```python
from build123d import *

# Parameters (mm, degrees)
SKETCH1_W           = 22.5
SKETCH1_H           = 12
BOSS_EXTRUDE1_DEPTH = 21
SKETCH2_W           = 32.5
SKETCH2_H           = 12
BOSS_EXTRUDE2_DEPTH = 3
SKETCH3_W           = 22.5
SKETCH3_H           = 12
BOSS_EXTRUDE6_DEPTH = 4
SKETCH5_W           = 12
SKETCH5_H           = 12
BOSS_EXTRUDE7_DEPTH = 5
SKETCH6_R           = 3.5
BOSS_EXTRUDE8_DEPTH = 5
SKETCH7_R           = 1.2
CUT_EXTRUDE1_DEPTH  = 5
FILLET3_R           = 3
FILLET4_R           = 1
FILLET5_R           = 1
FILLET6_R           = 1
FILLET7_R           = 1
FILLET8_R           = 1
FILLET9_R           = 1
FILLET10_R          = 0.2
SKETCH14_R          = 2.1
CUT_EXTRUDE4_DEPTH  = 5
SKETCH13_R          = 2.1
CUT_EXTRUDE5_DEPTH  = 5
FILLET11_R          = 1


with BuildPart() as part:
    # Sketch1 → Boss-Extrude1 (new body)
    with BuildSketch(Plane.XY):
        Rectangle(SKETCH1_W, SKETCH1_H)
    extrude(amount=BOSS_EXTRUDE1_DEPTH)

    # Sketch2 → Boss-Extrude2 (add)
    with BuildSketch(Plane.XY):
        Rectangle(SKETCH2_W, SKETCH2_H)
    extrude(amount=-BOSS_EXTRUDE2_DEPTH)

    # Sketch3 → Boss-Extrude6 (add)
    with BuildSketch(Plane(origin=(0, 0, -3), x_dir=(-1, 0, 0), z_dir=(0, 0, -1))):
        Rectangle(SKETCH3_W, SKETCH3_H)
    extrude(amount=BOSS_EXTRUDE6_DEPTH)

    # Sketch5 → Boss-Extrude7 (add)
    with BuildSketch(Plane(origin=(0, 0, -7), x_dir=(-1, 0, 0), z_dir=(0, 0, -1))):
        with Locations((-5.25, 0)):
            Rectangle(SKETCH5_W, SKETCH5_H)
    extrude(amount=BOSS_EXTRUDE7_DEPTH)

    # Sketch6 → Boss-Extrude8 (add)
    with BuildSketch(Plane(origin=(0, 0, -12), x_dir=(-1, 0, 0), z_dir=(0, 0, -1))):
        with Locations(Location((-5.25, 0, 0), (0, 0, 180))):
            Circle(SKETCH6_R)
    extrude(amount=BOSS_EXTRUDE8_DEPTH)

    # Sketch7 → Cut-Extrude1 (cut)
    with BuildSketch(Plane(origin=(0, 0, -17), x_dir=(-1, 0, 0), z_dir=(0, 0, -1))):
        with Locations((-5.25, 0)):
            Circle(SKETCH7_R)
    extrude(amount=-CUT_EXTRUDE1_DEPTH, mode=Mode.SUBTRACT)

    # Fillet3
    fillet3_edges = [part.edges().sort_by_distance(p)[0] for p in [
        (-11.25, 0, -7),
    ]]
    fillet(fillet3_edges, radius=FILLET3_R)

    # Fillet4
    fillet4_edges = [part.edges().sort_by_distance(p)[0] for p in [
        (11.25, 0, -12),
    ]]
    fillet(fillet4_edges, radius=FILLET4_R)

    # Fillet5
    fillet5_edges = [part.edges().sort_by_distance(p)[0] for p in [
        (-0.75, 0, -12),
    ]]
    fillet(fillet5_edges, radius=FILLET5_R)

    # Fillet6
    fillet6_edges = [part.edges().sort_by_distance(p)[0] for p in [
        (11.25, -6, -7),
        (10.957106781, -6, -11.707106781),
        (-0.75, -6, -9),
        (-0.457106781, -6, -11.707106781),
        (5.25, -6, -12),
    ]]
    fillet(fillet6_edges, radius=FILLET6_R)

    # Fillet7
    fillet7_edges = [part.edges().sort_by_distance(p)[0] for p in [
        (11.25, 6, -7),
        (10.957106781, 6, -11.707106781),
        (-0.75, 6, -9),
        (-0.457106781, 6, -11.707106781),
        (5.25, 6, -12),
    ]]
    fillet(fillet7_edges, radius=FILLET7_R)

    # Fillet8
    fillet8_edges = [part.edges().sort_by_distance(p)[0] for p in [
        (-11.25, 6, -3.5),
        (-10.371320344, 6, -6.121320344),
        (-4, 6, -7),
    ]]
    fillet(fillet8_edges, radius=FILLET8_R)

    # Fillet9
    fillet9_edges = [part.edges().sort_by_distance(p)[0] for p in [
        (-11.25, -6, -3.5),
        (-10.371320344, -6, -6.121320344),
        (-4, -6, -7),
    ]]
    fillet(fillet9_edges, radius=FILLET9_R)

    # Fillet10
    fillet10_edges = [part.edges().sort_by_distance(p)[0] for p in [
        (1.75, 0, -17),
    ]]
    fillet(fillet10_edges, radius=FILLET10_R)

    # Sketch14 → Cut-Extrude4 (cut)
    with BuildSketch(Plane(origin=(0, 0, -3), x_dir=(-1, 0, 0), z_dir=(0, 0, -1))):
        with Locations((15, 0)):
            Circle(SKETCH14_R)
    extrude(amount=-CUT_EXTRUDE4_DEPTH, mode=Mode.SUBTRACT)

    # Sketch13 → Cut-Extrude5 (cut)
    with BuildSketch(Plane(origin=(0, 0, -3), x_dir=(-1, 0, 0), z_dir=(0, 0, -1))):
        with Locations((-15, 0)):
            Circle(SKETCH13_R)
    extrude(amount=-CUT_EXTRUDE5_DEPTH, mode=Mode.SUBTRACT)

    # Fillet11
    fillet11_edges = [part.edges().sort_by_distance(p)[0] for p in [
        (-16.25, -6, -1.5),
        (-16.25, 6, -1.5),
        (16.25, -6, -1.5),
        (16.25, 6, -1.5),
    ]]
    fillet(fillet11_edges, radius=FILLET11_R)


solid = part.part
```
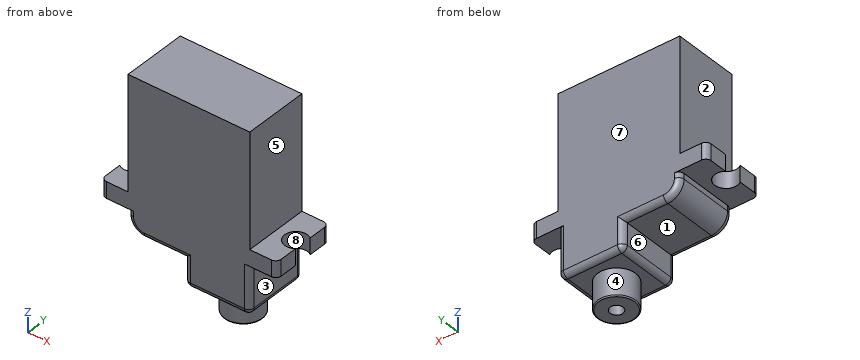
The listing builds one solid part. Answer for the finished solid, in the listing's coordinates (mm). Face numbers are marked on the shaded views. A direction names the side the tool comes from. Give positions to 0.01 mm unless a question says otherwise; leave off trailing zeros. Write each loop counter-clockwise with the first axis right and the second up, starting at its lowest first coordinate (ties: lowest second). Pieces come first, ordered by that corner, then holes. Notation, with made-up numbers: (-30.75, 40.25) -> (-19.75, 40.25) arc R18 ccw to (-19.75, 59.25) -> close; hole circle Ø3 at (45, -15). An arc over 180 degrees is marked (long way). Write item = value, one per line. Start each with the question number.
1) Straight lines are drawn through the part: line 1 along Y through (x, z) = (15, -0.9); line 2 along Z through (x, y) = (12.5, -3.25); line 3 along X through (y, z) = (0, -1.6). For each, find the intervals that lie inside material, in ascending order.
2) Each of these flat-tipped pins is pushed along its axis until it touches: pin 1 (1 mm diameter, centred on y = 1, z = 4.5, fed in from -X); pin 2 (6.5 mm diameter, centred on x = 13.5, y = 0, fed in from -Z); pin 3 (5 mm diameter, centred on x = -13, y = 2.5, fed in from -Z). Where does it stop, or does it pass through?
3) The part is cut by section D-D, the plane x = -5.5. Determine the outline of the cut face in (y, z).
4) The part is cut by section A-A, the plane x = 5.25. Determine the outline of the cut face in (y, z).
5) Which of the six approach directions +Z, -Z, +X, -X, +Y, -Y give full straight-line access (tool end or side, diameter ignored) to the marked faces 1, 2, 3, 4 and 5?
6) Determine the mould class of the marked faces 6, 7 and 8 for opening direction X: +X half, -X half, draft (parallel to the pull), parting line (faces both ways), or undercut.
7) The part is cut by section B-B, the plane y = 0. Determine the outline of the cut face in (x, z).
8) The part is cut by section C-C, the plane z = -8.5. Determine the outline of the cut face in (x, y).
Solutions:
q1.line_1 = -6 to -2.1, 2.1 to 6
q1.line_2 = -3 to 0
q1.line_3 = -12.9 to 12.9
q2.pin_1 = -11.25
q2.pin_2 = -12
q2.pin_3 = -5.98
q3.outline = (-6, -6) arc R1 ccw to (-5, -7) -> (5, -7) arc R1 ccw to (6, -6) -> (6, 21) -> (-6, 21) -> close
q4.outline = (-6, -11) arc R1 ccw to (-5, -12) -> (-3.5, -12) -> (-3.5, -16.8) arc R0.2 ccw to (-3.3, -17) -> (-1.2, -17) -> (-1.2, -12) -> (1.2, -12) -> (1.2, -17) -> (3.3, -17) arc R0.2 ccw to (3.5, -16.8) -> (3.5, -12) -> (5, -12) arc R1 ccw to (6, -11) -> (6, 21) -> (-6, 21) -> close
q5.face_1 = -Z, -X, +Y, -Y
q5.face_2 = +Z, -X, +Y, -Y
q5.face_3 = -Z, +X, +Y, -Y
q5.face_4 = -Z
q5.face_5 = +Z, +X, +Y, -Y
q6.face_6 = -X half
q6.face_7 = draft
q6.face_8 = undercut
q7.outline = (-12.9, -3) -> (-11.25, -3) -> (-11.25, -4) arc R3 ccw to (-8.25, -7) -> (-0.75, -7) -> (-0.75, -11) arc R1 ccw to (0.25, -12) -> (1.75, -12) -> (1.75, -16.8) arc R0.2 ccw to (1.95, -17) -> (4.05, -17) -> (4.05, -12) -> (6.45, -12) -> (6.45, -17) -> (8.55, -17) arc R0.2 ccw to (8.75, -16.8) -> (8.75, -12) -> (10.25, -12) arc R1 ccw to (11.25, -11) -> (11.25, -3) -> (12.9, -3) -> (12.9, 0) -> (11.25, 0) -> (11.25, 21) -> (-11.25, 21) -> (-11.25, 0) -> (-12.9, 0) -> close
q8.outline = (-0.75, -5) arc R1 ccw to (0.25, -6) -> (10.25, -6) arc R1 ccw to (11.25, -5) -> (11.25, 5) arc R1 ccw to (10.25, 6) -> (0.25, 6) arc R1 ccw to (-0.75, 5) -> close
